from build123d import *

# Parameters (mm, degrees)
F0_W     = 10
F0_H     = 1
F1_DEPTH = 1


with BuildPart() as f1:
    # F0 (on Top) → F1 (new body)
    with BuildSketch(Plane.XY):
        Polygon((10, 0), (0, 0), (0, -1), (0, -9), (0, -10), (10, -10), (10, -9), (10, -1), align=None)
        with Locations((-5, -0.5)):
            Rectangle(F0_W, F0_H)
        with Locations((15, -0.5)):
            Rectangle(F0_W, F0_H)
        with Locations((-5, -9.5)):
            Rectangle(F0_W, F0_H)
        with Locations((15, -9.5)):
            Rectangle(F0_W, F0_H)
    extrude(amount=F1_DEPTH)


solid = f1.part
The model under review builds one solid part; all positions refer to its coordinate system, in mm. A direction names the side the tool comes from. Give positions to 0.01 mm unless a question says otherwise; leave off trailing zeros. Order: outer loops, then holes, each group sorted by start corner. A loop starts at its lowest first (then second) coordinate and runs counter-clockwise, first axis right, second up. Notation, with made-up numbers: M 13.5,33.25 L 50.5,33.25 A8 cw 50.5,43.25 Z; hole C 81.25,58.5 d8. An arc over 180 degrees is marked long. Answer in a Markdown table with one row per item. Add a question column.
1. To check wall thickness, follow line 1 along Y through (x, z) = (13.5, 0.35); line 2 along X through (y, z) = (-2.5, 0.3). State the ranges of each line that lie inside material, in increasing order.
2. Add section A-A on x = 17.25. State the section outline as (y, z) points.
3. Machinability: for faces 4 (the flat face through (-5.1, -9, 0.5)), 5 (the flat face through (14.9, -9, 0.5)), 6 (the flat face through (5, -5, 1)), which of the approach directions +Z, -Z, +X, -X, +Y, -Y give a long, thin tool a straight path to every point of the face, cutting with its end or side? Answer none if there is none.
4. Add section B-B on z = 0.8. State the section outline as (x, y) points.
5. Mouldability with a two-part tool opening along Y and no side actions: class faces 1 (the flat face through (4.8, -10, 0.5)), 2 (the flat face through (-10, -9.5, 0.5)), 3 (the flat face through (10, -5.1, 0.5)) as released by +Y, released by -Y, zero draft, split by the parting line, or undercut.
6. Add section C-C on y = -6.5. State the section outline as (x, z) points, plus the area to 3 significant figures.
The answers:
| question | item | result |
|---|---|---|
| 1 | line 1 | -10 to -9, -1 to 0 |
| 1 | line 2 | 0 to 10 |
| 2 | outline | M -10,0 L -9,0 L -9,1 L -10,1 Z; M -1,0 L 0,0 L 0,1 L -1,1 Z |
| 3 | face 4 | +Z, -Z, -X |
| 3 | face 5 | +Z, -Z, +X |
| 3 | face 6 | +Z, +X, -X, +Y, -Y |
| 4 | outline | M -10,-10 L 20,-10 L 20,-9 L 10,-9 L 10,-1 L 20,-1 L 20,0 L -10,0 L -10,-1 L 0,-1 L 0,-9 L -10,-9 Z |
| 5 | face 1 | released by -Y |
| 5 | face 2 | zero draft |
| 5 | face 3 | undercut |
| 6 | outline | M 0,0 L 10,0 L 10,1 L 0,1 Z |
| 6 | area | 10.0 mm2 |
